```python
from build123d import *

# Parameters (mm, degrees)
ARM_DEPTH               = 6.35
CUT_EXTRUDE1_DEPTH      = 103.539993784
CUT_EXTRUDE1_DEPTH_BACK = 103.539993784
SKETCH2_R               = 1.27
CUT_EXTRUDE2_DEPTH      = 103.539993784
CUT_EXTRUDE2_DEPTH_BACK = 103.539993784
SKETCH3_R               = 1.27
FILLET1_R               = 2.54
FILLET2_R               = 6.35
FILLET3_R               = 6.35


# Some blends are built 0.0001 mm under size
with BuildPart() as part:
    # Sketch1 → Arm (new body)
    with BuildSketch(Plane(origin=(0, 0, 0), x_dir=(1, 0, 0), z_dir=(0, 1, 0))):
        Polygon((0, -18.5), (69.52, -15.430656357), (69.80008291, -21.774476465), (82.50008291, -21.213764954), (82.22, -14.869944846), (100, -14.08494873), (100, -9), (87.3, -9.560711511), (87.3, 9.560711511), (100, 9), (100, 14.08494873), (0, 18.5), (0, 13.41505127), (15.24, 12.742197457), (15.24, -12.742197457), (0, -13.41505127), align=None)
        Polygon((82.22, -9.784996116), (52.54, -11.095383333), (52.54, 11.095383333), (82.22, 9.784996116), align=None, mode=Mode.SUBTRACT)
        Polygon((20.32, 12.517912852), (20.32, -12.517912852), (47.46, -11.319667937), (47.46, 11.319667937), align=None, mode=Mode.SUBTRACT)
    extrude(amount=ARM_DEPTH)

    # Sketch2 → Cut-Extrude1 (cut, two sides: drawn at the far end of the back side and taken through both)
    with BuildSketch(Plane.XY.offset(-CUT_EXTRUDE1_DEPTH_BACK)):
        with Locations(Location((76.2, 3.175, 0), (0, 0, 180))):
            Circle(SKETCH2_R)
    extrude(amount=CUT_EXTRUDE1_DEPTH + CUT_EXTRUDE1_DEPTH_BACK, mode=Mode.SUBTRACT)

    # Sketch3 → Cut-Extrude2 (cut, two sides: drawn at the far end of the back side and taken through both)
    with BuildSketch(Plane.XY.offset(-CUT_EXTRUDE2_DEPTH_BACK)):
        with Locations((96.19, 3.175)):
            Circle(SKETCH3_R)
        with Locations(Location((3.81, 3.175, 0), (0, 0, 180))):
            Circle(SKETCH3_R)
    extrude(amount=CUT_EXTRUDE2_DEPTH + CUT_EXTRUDE2_DEPTH_BACK, mode=Mode.SUBTRACT)

    # Fillet1
    fillet1_edges = [part.edges().sort_by_distance(p)[0] for p in [
        (0, 0, -15.957525635),
        (100, 0, -11.542474365),
        (100, 0, 11.542474365),
        (0, 0, 15.957525635),
        (100, 6.35, 11.542474365),
        (100, 6.35, -11.542474365),
        (0, 6.35, 15.957525635),
        (0, 6.35, -15.957525635),
    ]]
    fillet(fillet1_edges, radius=FILLET1_R)

    # Fillet2
    # the kernel refuses this fillet: 6.35 mm, written as the material it adds along each edge
    with BuildSketch(Plane(origin=(15.24, 0, 12.742197457), x_dir=(-0.999026788670257, 0, 0.04410754492367402), z_dir=(0, 1, 0)), Plane(origin=(15.24, 0, -12.742197457), x_dir=(0, 0, 1), z_dir=(0, 1, 0))) as fillet2_piece_1:
        with BuildLine():
            CenterArc((FILLET2_R * 0.95682364669, -FILLET2_R), FILLET2_R, 90, 87.472003686)
            Line((-FILLET2_R * 0.0422031419804, -FILLET2_R * 0.955892455076), (0, 0))
            Line((0, 0), (FILLET2_R * 0.95682364669, 0))
        make_face()
    extrude(amount=6.35)
    with BuildSketch(Plane(origin=(87.3, 0, 9.560711511), x_dir=(0.9990267886702568, 0, -0.04410754492367471), z_dir=(0, 1, 0)), Plane(origin=(52.54, 0, 11.095383333), x_dir=(0.9990267886702568, 0, -0.044107544923674566), z_dir=(0, 1, 0)), Plane(origin=(20.32, 0, 12.517912852), x_dir=(0.9990267886702568, 0, -0.044107544923674614), z_dir=(0, 1, 0)), Plane(origin=(87.3, 0, -9.560711511), x_dir=(0, 0, 1), z_dir=(0, 1, 0)), Plane(origin=(52.54, 0, -11.095383333), x_dir=(0, 0, 1), z_dir=(0, 1, 0))) as fillet2_piece_2:
        with BuildLine():
            CenterArc((FILLET2_R * 1.0451246721, FILLET2_R), FILLET2_R, 177.472003686, 92.527996314)
            Line((FILLET2_R * 0.0460978834253, FILLET2_R * 1.04410754492), (0, 0))
            Line((0, 0), (FILLET2_R * 1.0451246721, 0))
        make_face()
    extrude(amount=6.35)
    with BuildSketch(Plane(origin=(47.46, 0, 11.319667937), x_dir=(0, 0, -1), z_dir=(0, 1, 0)), Plane(origin=(47.46, 0, -11.319667937), x_dir=(-0.9990267886702568, 0, -0.04410754492367462), z_dir=(0, 1, 0))) as fillet2_piece_3:
        with BuildLine():
            CenterArc((FILLET2_R * 0.95682364669, FILLET2_R), FILLET2_R, 182.527996314, 87.472003686)
            Line((-FILLET2_R * 0.0422031419804, FILLET2_R * 0.955892455076), (0, 0))
            Line((0, 0), (FILLET2_R * 0.95682364669, 0))
        make_face()
    extrude(amount=6.35)
    with BuildSketch(Plane(origin=(20.32, 0, -12.517912852), x_dir=(0.9990267886702568, 0, 0.044107544923674594), z_dir=(0, 1, 0))) as fillet2_piece_4:
        with BuildLine():
            CenterArc((FILLET2_R * 1.0451246721, -FILLET2_R), FILLET2_R, 90, 92.527996314)
            Line((FILLET2_R * 0.0460978834253, -FILLET2_R * 1.04410754492), (0, 0))
            Line((0, 0), (FILLET2_R * 1.0451246721, 0))
        make_face()
    extrude(amount=6.35)
    with BuildSketch(Plane(origin=(82.22, 0, 9.784996116), x_dir=(-0.9990267886702568, 0, 0.04410754492367457), z_dir=(0, 1, 0))) as fillet2_piece_5_section:
        with BuildLine():
            CenterArc((FILLET2_R * 0.95682364669, -FILLET2_R), FILLET2_R, 90, 87.472003686)
            Line((-FILLET2_R * 0.0422031419804, -FILLET2_R * 0.955892455076), (0, 0))
            Line((0, 0), (FILLET2_R * 0.95682364669, 0))
        make_face()
    fillet2_piece_5 = extrude(amount=6.35, mode=Mode.PRIVATE)
    fillet2_piece_5 = fillet2_piece_5 - Plane(origin=(76.2, 3.175, 9.784996116), x_dir=(-1, 0, 0), z_dir=(0, 0, -1)) * Cylinder(1.27, 38, mode=Mode.PRIVATE)
    add(fillet2_piece_5)
    with BuildSketch(Plane(origin=(82.22, 0, -9.784996116), x_dir=(-0.9990267886702568, 0, -0.04410754492367478), z_dir=(0, 1, 0))) as fillet2_piece_6_section:
        with BuildLine():
            CenterArc((FILLET2_R * 0.95682364669, FILLET2_R), FILLET2_R, 182.527996314, 87.472003686)
            Line((-FILLET2_R * 0.0422031419804, FILLET2_R * 0.955892455076), (0, 0))
            Line((0, 0), (FILLET2_R * 0.95682364669, 0))
        make_face()
    fillet2_piece_6 = extrude(amount=6.35, mode=Mode.PRIVATE)
    fillet2_piece_6 = fillet2_piece_6 - Plane(origin=(76.2, 3.175, -9.784996116), x_dir=(-1, 0, 0), z_dir=(0, 0, 1)) * Cylinder(1.27, 38, mode=Mode.PRIVATE)
    add(fillet2_piece_6)

    # Fillet3
    fillet3_edges = [part.edges().sort_by_distance(p)[0] for p in [
        (69.52, 3.175, 15.430656357),
        (82.22, 3.175, 14.869944846),
    ]]
    fillet(fillet3_edges, radius=FILLET3_R - 0.0001)  # a hair under: the kernel refuses the full size


solid = part.part
```
Here's how the part is built. I have some questions about the finished solid (model axes, mm). A direction names the side the tool comes from. Round coordinates to 2 decimals unless told otherwise and drop trailing zeros. Order: outer loops, then holes, each group sorted by start corner. A loop starts at its lowest first (then second) coordinate and runs counter-clockwise, first axis right, second up. Notation, with made-up numbers: M -4.75,-12 L 22.25,-12 A20 cw 22.25,25 Z; hole C 62.25,52 d3. An arc over 180 degrees is marked long. One line per question, with ' | ' between items.
1) For faces 5 (the face through (74.99, 2.79, -12.56)), 6 (the face through (13.52, 3.13, -11.01)), 7 (the face through (97.7, 3.1, 9.1)), which set-ups out of +Z, -Z, +X, -X, +Y, -Y let a thin tool reach every point of the face, with its end or its side?
Working result:
face 5: +Z, -Z | face 6: -X, +Y, -Y | face 7: +Y, -Y
2) I want a section at D-D, the plane x = 14. Write out the boundary of the cut face in (y, z).
Working result:
outline: M 0,-17.88 L 6.35,-17.88 L 6.35,-10.44 L 0,-10.44 Z; M 0,10.44 L 6.35,10.44 L 6.35,17.88 L 0,17.88 Z
3) I want a section at A-A, the plane z = 17.5. Write out the boundary of the cut face in (x, y) (3 decimals), then the cut area to 3 significant figures.
Working result:
outline: M 0,2.54 A2.54 ccw 2.54,0 L 22.65,0 L 22.65,6.35 L 2.54,6.35 A2.54 ccw 0,3.81 Z; M 67.881,0 L 83.502,0 L 83.502,6.35 L 67.881,6.35 Z; hole C 3.81,3.175 d2.54; hole C 76.2,3.175 d2.54 | area: 230 mm²
4) I want a section at C-C, the plane x = 3.81. Write out the boundary of the cut face in (y, z) (3 decimals), then the cut area to 3 significant figures.
Working result:
outline: M 0,-18.332 L 1.905,-18.332 L 1.905,-13.247 L 0,-13.247 Z; M 0,13.247 L 1.905,13.247 L 1.905,18.332 L 0,18.332 Z; M 4.445,-18.332 L 6.35,-18.332 L 6.35,-13.247 L 4.445,-13.247 Z; M 4.445,13.247 L 6.35,13.247 L 6.35,18.332 L 4.445,18.332 Z | area: 38.7 mm²
5) I need wall thicknesses on line 1 along X through (y, z) = (5.5, -1.5); line 2 along X through (y, z) = (3.25, 13.5); line 3 along Y through (x, z) = (96, -12). Which ranges of each line are inside material? Lowest first, please.
Working result:
line 1: 15.24 to 20.32, 47.46 to 52.54, 82.22 to 87.3 | line 2: 0 to 2.54, 5.08 to 74.93, 77.47 to 94.92, 97.46 to 100 | line 3: 0 to 1.92, 4.43 to 6.35
6) For pin 1 Ø1.9 at (y, z) = (3.5, 2) entering from -X; pin 2 Ø1.5 at (x, y) = (96.19, 3.175) entering from -Z; pin 3 Ø3 at (y, z) = (3.5, 1.5) entering from +X; pin 4 Ø1.5 at (y, z) = (2.5, 8) entering from -X, each with a flat end and sliding along its axis, tell me the tip position at first contact or that it passes through.
Working result:
pin 1: x = 15.24 | pin 2: through | pin 3: x = 87.3 | pin 4: x = 14.89
7) I want a section at B-B, the plane x = 56. Write out the boundary of the cut face in (y, z).
Working result:
outline: M 0,-16.03 L 6.35,-16.03 L 6.35,-10.11 L 0,-10.11 Z; M 0,10.11 L 6.35,10.11 L 6.35,16.03 L 0,16.03 Z
8) If we mould it in two halves opening along X, with no side actions, what happens to faces 1 (the face through (15.24, 3, 0)), 2 (the face through (99.236, 5.626, 11.562)), 3 (the face through (31.146, 3.131, 17.125)), 4 (the face through (49, 0, 3))? For each: +X half, -X half, draft (parallel to the pull), parting line (faces both ways), or undercut.
Working result:
face 1: -X half | face 2: +X half | face 3: undercut | face 4: draft
